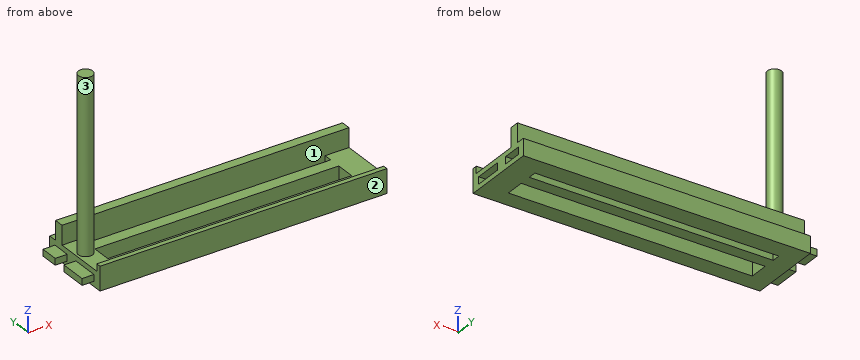
from build123d import *

# Parameters (mm, degrees)
SKETCH1_W               = 120
SKETCH1_H               = 31.25
BOSS_EXTRUDE1_DEPTH     = 7
SKETCH2_W               = 120
SKETCH2_H               = 4
SKETCH2_H_2             = 2
BOSS_EXTRUDE2_DEPTH     = 8
CUT_EXTRUDE1_DEPTH      = 125.260059955
CUT_EXTRUDE1_DEPTH_BACK = 125.260059955
SKETCH3_W               = 102
SKETCH3_H               = 8
SKETCH3_H_2             = 3.5
SKETCH4_W               = 2.75
SKETCH4_H               = 7.59061182
SKETCH4_H_2             = 11.2
BOSS_EXTRUDE3_DEPTH     = 5
SKETCH5_W               = 3
SKETCH5_H               = 8.0580149
SKETCH5_H_2             = 11.6919851
CUT_EXTRUDE2_DEPTH      = 5
CUT_EXTRUDE3_REACH      = 126.906
SKETCH6_W               = 5
SKETCH6_H               = 2
SKETCH7_R               = 3
BOSS_EXTRUDE4_DEPTH     = 72


with BuildPart() as part:
    # Sketch1 → Boss-Extrude1 (new body)
    with BuildSketch(Plane.XY):
        with Locations((60, 15.625)):
            Rectangle(SKETCH1_W, SKETCH1_H)
    extrude(amount=BOSS_EXTRUDE1_DEPTH)

    # Sketch2 → Boss-Extrude2 (add)
    with BuildSketch(Plane.XY.offset(7)):
        with Locations((60, 25.6)):
            Rectangle(SKETCH2_W, SKETCH2_H)
        with Locations((60, 1)):
            Rectangle(SKETCH2_W, SKETCH2_H_2)
    extrude(amount=BOSS_EXTRUDE2_DEPTH)

    # Sketch3 → Cut-Extrude1 (cut, two sides: drawn at the far end of the back side and taken through both)
    with BuildSketch(Plane.XY.offset(7).offset(-CUT_EXTRUDE1_DEPTH_BACK)):
        with Locations((59, 11.1)):
            Rectangle(SKETCH3_W, SKETCH3_H)
        with Locations((59, 21.85)):
            Rectangle(SKETCH3_W, SKETCH3_H_2)
    extrude(amount=CUT_EXTRUDE1_DEPTH + CUT_EXTRUDE1_DEPTH_BACK, mode=Mode.SUBTRACT)

    # Sketch4 → Boss-Extrude3 (add)
    with BuildSketch(Plane.ZY):
        with Locations((3.5, 24.20469409)):
            Rectangle(SKETCH4_W, SKETCH4_H)
        with Locations((3.5, 9.35)):
            Rectangle(SKETCH4_W, SKETCH4_H_2)
    extrude(amount=BOSS_EXTRUDE3_DEPTH)

    # Sketch5 → Cut-Extrude2 (cut)
    with BuildSketch(Plane(origin=(120, 0, 0), x_dir=(0, 0, -1), z_dir=(1, 0, 0))):
        with Locations((-3.5, 24.22099255)):
            Rectangle(SKETCH5_W, SKETCH5_H)
        with Locations((-3.5, 9.34599255)):
            Rectangle(SKETCH5_W, SKETCH5_H_2)
    extrude(amount=-CUT_EXTRUDE2_DEPTH, mode=Mode.SUBTRACT)

    # Sketch6 → Cut-Extrude3 (cut, up to next)
    with BuildSketch(Plane.ZY, mode=Mode.PRIVATE) as cut_extrude3_sk1:
        with Locations((12.5, 1)):
            Rectangle(SKETCH6_W, SKETCH6_H)
    cut_extrude3_tool1 = extrude(cut_extrude3_sk1.sketch, amount=-CUT_EXTRUDE3_REACH, mode=Mode.PRIVATE) & part.part
    add(cut_extrude3_tool1.solids().sort_by_distance((0, 1, 12.5))[0], mode=Mode.SUBTRACT)

    # Sketch7 → Boss-Extrude4 (add)
    with BuildSketch(Plane.XY.offset(7)):
        with Locations(Location((4, 14.95, 0), (0, 0, 180))):
            Circle(SKETCH7_R)
    extrude(amount=BOSS_EXTRUDE4_DEPTH)


solid = part.part
For this review, take the finished solid that the model builds, in its own axes (mm). Face numbers are marked on the shaded views. Round coordinates to 2 decimals unless told otherwise and drop trailing zeros. Order: outer loops, then holes, each group sorted by start corner. A loop starts at its lowest first (then second) coordinate and runs counter-clockwise, first axis right, second up. Notation, with made-up numbers: M -9,19 L 33,19 A23 cw 33,49 Z; hole C 27.5,16.25 d5. An arc over 180 degrees is marked long. Use a Markdown table: item, result. Add a question column.
Item 1: Add section C-C, the plane x = 4. Give the boundary of the cut face in (y, z).
Item 2: Add section D-D, the plane z = 43. Give the boundary of the cut face in (x, y).
Item 3: Mouldability with a two-part tool opening along X and no side actions: class the marked faces 1, 2 and 3 as released by +X, released by -X, zero draft, split by the parting line, or undercut.
Item 4: Add section A-A, the plane x = 19. Give the boundary of the cut face in (y, z).
Item 5: To check wall thickness, follow line 1 along Y through (x, z) = (22, 3); line 2 along Z through (x, y) = (80.5, 19); line 3 along Z through (x, y) = (4, 24). State the ranges of each line that lie inside material, in increasing order.
Item 6: Add section B-B, the plane y = 13.5. Give the boundary of the cut face in (x, z) (3 decimals).
Item 7: Insertion check: pin 1 (2.5 mm diameter, centred on x = 118, y = 9.5, fed in from +Z); pin 2 (2.5 mm diameter, centred on x = -2.5, y = 8, fed in from -Z) (3 decimals); pin 3 (1.4 mm diameter, centred on x = -2.5, z = 3, fed in from -Y). Each pin has a flat end and moves straight along its axis. Give the tip position at first contact, or say it passes through.
Geometry results:
| question | item | result |
|---|---|---|
| 1 | outline | M 0,0 L 31.25,0 L 31.25,7 L 27.6,7 L 27.6,15 L 23.6,15 L 23.6,7 L 17.95,7 L 17.95,79 L 11.95,79 L 11.95,7 L 2,7 L 2,10 L 0,10 Z |
| 2 | outline | C 4,14.95 d6 |
| 3 | face 1 | undercut |
| 3 | face 2 | zero draft |
| 3 | face 3 | split by the parting line |
| 4 | outline | M 0,0 L 7.1,0 L 7.1,7 L 2,7 L 2,10 L 0,10 Z; M 15.1,0 L 20.1,0 L 20.1,7 L 15.1,7 Z; M 23.6,0 L 31.25,0 L 31.25,7 L 27.6,7 L 27.6,15 L 23.6,15 Z |
| 5 | line 1 | y = 0 to 7.1, 15.1 to 20.1, 23.6 to 31.25 |
| 5 | line 2 | z = 0 to 7 |
| 5 | line 3 | z = 0 to 15 |
| 6 | outline | M -5,2.125 L 0,2.125 L 0,0 L 8,0 L 8,7 L 6.626,7 L 6.626,79 L 1.374,79 L 1.374,7 L 0,7 L 0,4.875 L -5,4.875 Z; M 110,0 L 120,0 L 120,2 L 115,2 L 115,5 L 120,5 L 120,7 L 110,7 Z |
| 7 | pin 1 | stops at z = 7 |
| 7 | pin 2 | stops at z = 2.125 |
| 7 | pin 3 | stops at y = 3.75 |
